Answer from the drawing. Dimensions are ordinates in mm from the lowest x, y and z of the part. A direction names the side the tool comes from. Give positions to 0.01 mm unless a question says otherwise; leave off trailing zeros. Write each loop counter-clockwise with the first axis right and the second up, starting at its lowest first coordinate (ties: lowest second). Pieces come first, ordered by that corner, then holes.
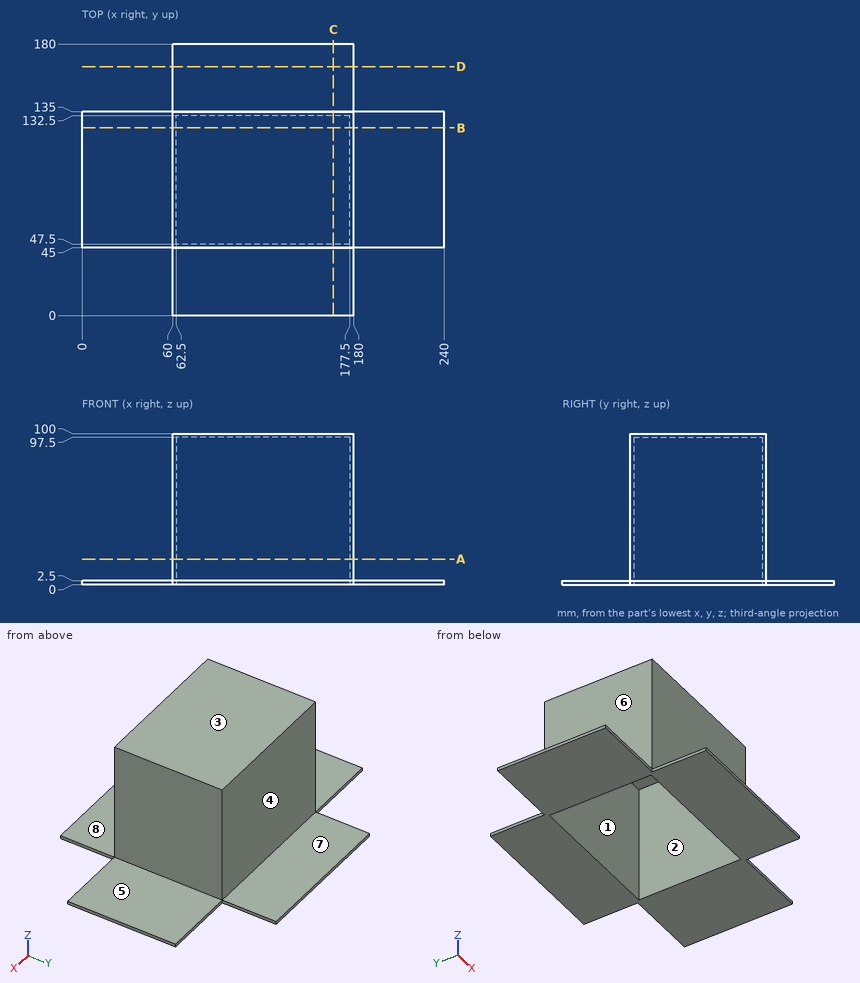
Item 1: Section B-B (y = 124.5) is taken. Write down the section's boundary in (x, z), and give its area (3 significant figures).
Result set:
outline: (0, 0) - (62.5, 0) - (62.5, 97.5) - (177.5, 97.5) - (177.5, 0) - (240, 0) - (240, 2.5) - (180, 2.5) - (180, 100) - (60, 100) - (60, 2.5) - (0, 2.5) - close
area: 1,090 mm2
Item 2: Each of these flat-tipped pins is pushed along its axis until it touches: pin 1 Ø1.5 at (y, z) = (52.5, 71) entering from -X; pin 2 Ø2 at (x, z) = (20, 1) entering from +Y; pin 3 Ø2 at (y, z) = (168.5, 1) entering from +X. Where does it stop, or does it pass through?
Result set:
pin 1: stops at x = 60
pin 2: stops at y = 135
pin 3: stops at x = 180
Item 3: Find the intervals of material crossed by line 1 along X through (y, z) = (57.5, 78); line 2 along Y through (x, z) = (107, 24.5); line 3 along Z through (x, y) = (201.5, 101.5), in increasing order.
Result set:
line 1: x = 60 to 62.5, 177.5 to 180
line 2: y = 45 to 47.5, 132.5 to 135
line 3: z = 0 to 2.5
Item 4: Which of the six approach directions +Z, -Z, +X, -X, +Y, -Y give full straight-line access (tool end or side, diameter ignored) to the marked faces 5, 6, 7 and 8?
Result set:
face 5: +Z, +X, +Y, -Y
face 6: +Z, -X, +Y, -Y
face 7: +Z, +X, -X, +Y
face 8: +Z, +X, -X, -Y
Item 5: Determine the mould class of the marked faces 1, 2, 3 and 4 for opening direction Y: pulls with the +Y half, pulls with the -Y half, needs draft (parallel to the pull), parting line crosses it, or undercut.
Result set:
face 1: undercut
face 2: undercut
face 3: needs draft
face 4: pulls with the +Y half
Item 6: Section D-D (y = 165) is taken. Write down the section's boundary in (x, z), and give its area (3 significant figures).
Result set:
outline: (60, 0) - (180, 0) - (180, 2.5) - (60, 2.5) - close
area: 300 mm2
Item 7: Section C-C (x = 166.5) is taken. Write down the section's boundary in (y, z), and give its area (4 significant figures).
Result set:
outline: (0, 0) - (47.5, 0) - (47.5, 97.5) - (132.5, 97.5) - (132.5, 0) - (180, 0) - (180, 2.5) - (135, 2.5) - (135, 100) - (45, 100) - (45, 2.5) - (0, 2.5) - close
area: 937.5 mm2
Item 8: Section A-A (z = 17) is taken. Write down the section's boundary in (x, y), and give its area (4 significant figures).
Result set:
outline: (60, 45) - (180, 45) - (180, 135) - (60, 135) - close; hole (62.5, 47.5) - (177.5, 47.5) - (177.5, 132.5) - (62.5, 132.5) - close
area: 1,025 mm2
